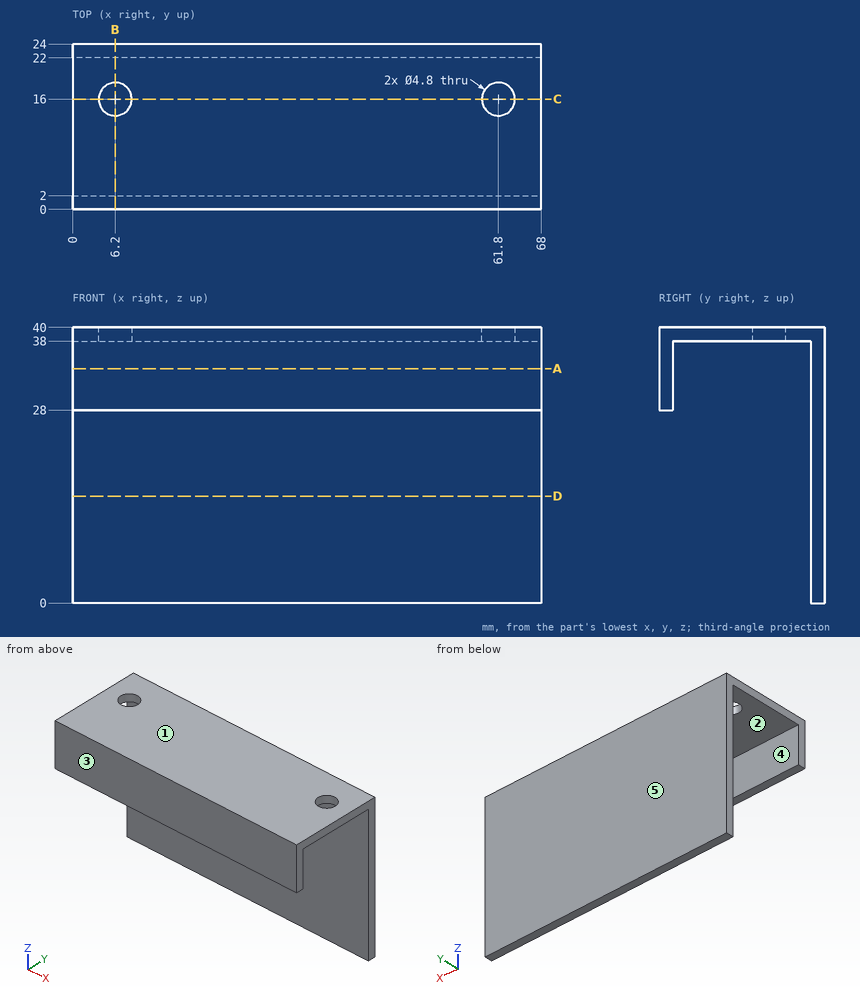
Study the drawing (mm; zero at the part's minimum x, y, z) and answer. A direction names the side the tool comes from. Round coordinates to 2 decimals unless told otherwise and drop trailing zeros. Loops run counter-clockwise (first coordinate to the right, second up) from the corner with the lowest first, then second, coordinate; pieces in that order, holes last. Notation, with made-up numbers: (-32, -30) -> (-18, -30) arc R14 cw to (-18, -9) -> close; hole circle Ø11 at (39.5, -14.75). An arc over 180 degrees is marked (long way). One line per item, written item: value.
1) The mould has two halves that part along Y. Classify the marked faces 3, 4 and 5: pulls with the +Y half, pulls with the -Y half, needs draft (parallel to the pull), parting line crosses it, or undercut.
Answer list:
face 3: pulls with the -Y half
face 4: undercut
face 5: pulls with the +Y half
2) A cutting plane is placed at B-B (x = 6.2). Determine the outline of the cut face in (y, z), and give its area (3 significant figures).
Answer list:
outline: (0, 28) -> (2, 28) -> (2, 38) -> (13.6, 38) -> (13.6, 40) -> (0, 40) -> close; (18.4, 38) -> (22, 38) -> (22, 0) -> (24, 0) -> (24, 40) -> (18.4, 40) -> close
area: 134 mm²
3) A cutting plane is placed at D-D (z = 15.5). Determine the outline of the cut face in (x, y).
Answer list:
outline: (0, 22) -> (68, 22) -> (68, 24) -> (0, 24) -> close
4) For the marked faces 1 and 2, determine the directions among +Z, -Z, +X, -X, +Y, -Y from which every point of the face is accessible in a straight line to the end or side of a thin tool.
Answer list:
face 1: +Z, +X, -X, +Y, -Y
face 2: -Z, +X, -X
5) Consider L1, parallel to Y at x = 6.2, z = 39.6; L2, parallel to Y at x = 22, z = 33.5; L3, parallel to Z at x = 27.5, y = 6.5. Determine where each line is inside the solid, lowest interval first. Write a range as [from, to].
Answer list:
L1: y = [0, 13.6], [18.4, 24]
L2: y = [0, 2], [22, 24]
L3: z = [38, 40]
6) Flat-ended cylindrical pins translate along their axes: P1, Ø4, axis at y = 14.5, z = 35, coming from the -X side; P2, Ø6, axis at x = 24, y = 14.5, coming from the -Z side; P3, Ø1, axis at x = 21.5, y = 1.5, coming from the -Z side; P4, Ø19, axis at x = 45.5, z = 13.5, coming from the -Y side. Find the tip coordinate at first contact, or state that the pin passes through.
Answer list:
P1: passes through
P2: stops at z = 38
P3: stops at z = 28
P4: stops at y = 22
7) A cutting plane is placed at A-A (z = 34). Determine the outline of the cut face in (x, y), and give its area (3 significant figures).
Answer list:
outline: (0, 0) -> (68, 0) -> (68, 2) -> (0, 2) -> close; (0, 22) -> (68, 22) -> (68, 24) -> (0, 24) -> close
area: 272 mm²
8) A cutting plane is placed at C-C (y = 16). Determine the outline of the cut face in (x, z), and give its area (3 significant figures).
Answer list:
outline: (0, 38) -> (3.8, 38) -> (3.8, 40) -> (0, 40) -> close; (8.6, 38) -> (59.4, 38) -> (59.4, 40) -> (8.6, 40) -> close; (64.2, 38) -> (68, 38) -> (68, 40) -> (64.2, 40) -> close
area: 117 mm²
